from build123d import *

# Parameters (mm, degrees)
F0_R     = 8.25
F1_DEPTH = 5
F2_R     = 6
F3_DEPTH = 5
F4_R     = 8.25
F5_DEPTH = 5


with BuildPart() as f1:
    # F0 (on Top) → F1 (new body)
    with BuildSketch(Plane.XY):
        Circle(F0_R)
    extrude(amount=-F1_DEPTH)

    # F2 (on Top) → F3 (join)
    with BuildSketch(Plane.XY):
        Circle(F2_R)
    extrude(amount=F3_DEPTH)

    # F4 (on face) → F5 (join)
    with BuildSketch(Plane.XY.offset(5)):
        Circle(F4_R)
    extrude(amount=F5_DEPTH)


solid = f1.part
Geometry: final body of the model. Coordinates: model frame, mm. A direction names the side the tool comes from. Give positions to 0.01 mm unless a question says otherwise; leave off trailing zeros. Order: outer loops, then holes, each group sorted by start corner. A loop starts at its lowest first (then second) coordinate and runs counter-clockwise, first axis right, second up. Notation, with made-up numbers: (46.25, 80.25) -> (78.25, 80.25) arc R26 cw to (78.25, 114.25) -> close; hole circle Ø11 at (53.25, 22.5). An arc over 180 degrees is marked (long way). Put each result on its own line as item: value.
Q1. Section A-A, the plane y = 0. Return loops of the section in (x, z).
Here are the results:
outline: (-8.25, -5) -> (8.25, -5) -> (8.25, 0) -> (6, 0) -> (6, 5) -> (8.25, 5) -> (8.25, 10) -> (-8.25, 10) -> (-8.25, 5) -> (-6, 5) -> (-6, 0) -> (-8.25, 0) -> close
Q2. Reachability of faces 4 (the face through (4, -5, 0)), 5 (the face through (7.62, -3.16, 7.46)) from +Z, -Z, +X, -X, +Y, -Y: full face, straight path, thin tool, end or side. Return the list, or none.
Here are the results:
face 4: none
face 5: +Z, -Z
Q3. Section C-C, the plane z = 0.5. Return loops of the section in (x, y).
Here are the results:
outline: circle Ø12 at (0, 0)
Q4. Draft query along Z for faces 1 (the face through (0, 0, 10)), 2 (the face through (4, -5, 5)), 3 (the face through (7.62, -3.16, -2.46)). Return one class per face: released by +Z, released by -Z, zero draft, split by the parting line, or undercut.
Here are the results:
face 1: released by +Z
face 2: undercut
face 3: zero draft
Q5. Material intervals for L1, parallel to Z at x = -0.5, y = -7.5; L2, parallel to Y at x = -0.25, z = -3.25; L3, parallel to X at y = 0.25, z = 0.75, sorted ascending.
Here are the results:
L1: z = -5 to 0, 5 to 10
L2: y = -8.25 to 8.25
L3: x = -5.99 to 5.99
Q6. Pin query (flat end, axial travel): pin 1 (1 mm diameter, centred on x = 3.5, z = 3, fed in from -Y); pin 2 (5 mm diameter, centred on x = 2, z = 2, fed in from -Y); pin 3 (1 mm diameter, centred on y = -1, z = 6.5, fed in from +X); pin 4 (8 mm diameter, centred on x = 2.5, z = 8, fed in from +Y). Return the tip coordinate at first contact, or that it passes through.
Here are the results:
pin 1: stops at y = -5.2
pin 2: stops at y = -8.23
pin 3: stops at x = 8.23
pin 4: stops at y = 8.25
